Input: part model. Units: mm. Frame: model coordinates. A direction names the side the tool comes from. Round coordinates to 2 decimals unless told otherwise and drop trailing zeros. Loops run counter-clockwise (first coordinate to the right, second up) from the corner with the lowest first, then second, coordinate; pieces in that order, holes last. Notation, with made-up numbers: (-29, 36.5) - (-2, 36.5) arc R30 ccw to (-2, 58.5) - close; hole circle Ø6 at (82.5, 34.5). An arc over 180 degrees is marked (long way). One line per question, with ' | ' between items. Start each with the question number.
Item 1: Draft query along X for faces 4 (the face through (20, 23.85, -20)), 5 (the face through (-12.5, 14, 0)), 6 (the face through (18.134, 13.942, -35.15)). Return one class per face: pulls with the +X half, pulls with the -X half, needs draft (parallel to the pull), parting line crosses it, or undercut.
Item 2: Set-up query: faces 1 (the face through (0, 23.85, 0)), 2 (the face through (26.812, 13.609, -12.528)), 3 (the face through (13, 14, -12)). Return all of +Z, -Z, +X, -X, +Y, -Y with unobstructed straight access to the full face (end or side cutting, diameter ignored); none if empty.
Item 3: First-contact query: pin 1 (6 mm diameter, centred on x = 1.5, z = -1, fed in from -Y); pin 2 (6 mm diameter, centred on y = 16, z = -17.5, fed in from -X); pin 3 (12 mm diameter, centred on x = 23.5, y = 23.5, fed in from +Z). Flat tips, straight axial feed; report the tip coordinate or a pass-through.
Item 4: Section B-B, the plane x = -3. Return loops of the section in (y, z), plus the area to 3 significant figures.
Item 5: Section A-A, the plane y = 15.75. Return loops of the section in (x, z), plus the area to 3 significant figures.
Item 6: Section D-D, the plane z = -11.5. Return loops of the section in (x, y).
Item 7: Section C-C, the plane z = -1.5. Return loops of the section in (x, y).
Item 8: Material intervals for line 1 along Z through (x, y) = (8.5, 5.75); line 2 along X through (y, z) = (18.25, -6); line 3 along X through (y, z) = (7.75, 2), sorted ascending.
```python
from build123d import *

# Parameters (mm, degrees)
SKETCH_1_W           = 25
SKETCH_1_H           = 25
SKETCH_1_W_2         = 20.2
SKETCH_1_H_2         = 20.2
EXTRUDE_1_DEPTH      = 20
SKETCH_2_W           = 25
SKETCH_2_H           = 25
EXTRUDE_2_DEPTH      = 7.5
EXTRUDE_3_DEPTH      = 17.67767
EXTRUDE_3_DEPTH_BACK = 20
SKETCH_3_W           = 35.35533906
SKETCH_3_H           = 27.5
SKETCH_3_W_2         = 20.2
SKETCH_3_H_2         = 20.2
SKETCH_1_3_W         = 20.2
SKETCH_1_3_H         = 20.2
CUT_EXTRUDE_1_DEPTH  = 23.85
SKETCH_3_2_W         = 20.2
SKETCH_3_2_H         = 20.2
CUT_EXTRUDE_2_DEPTH  = 20
EXTRUDE_4_REACH      = 62.275


with BuildPart() as part:
    # 스케치1 → 보스-돌출1 (new body)
    with BuildSketch(Plane(origin=(0, 0, 0), x_dir=(1, 0, 0), z_dir=(0, 1, 0))):
        Rectangle(SKETCH_1_W, SKETCH_1_H)
        Rectangle(SKETCH_1_W_2, SKETCH_1_H_2, mode=Mode.SUBTRACT)
    extrude(amount=EXTRUDE_1_DEPTH)

    # 스케치2 → 보스-돌출2 (add)
    with BuildSketch(Plane(origin=(0, 20, 0), x_dir=(1, 0, 0), z_dir=(0, 1, 0))):
        Rectangle(SKETCH_2_W, SKETCH_2_H)
    extrude(amount=EXTRUDE_2_DEPTH)

    # 스케치3 → 보스-돌출3 (add, two sides: drawn at the far end of the back side and taken through both)
    with BuildSketch(Plane(origin=(12.5, 0, -12.5), x_dir=(0.7071067811865476, 0, 0.7071067811865476), z_dir=(-0.7071067811865476, 0, 0.7071067811865476)).offset(-EXTRUDE_3_DEPTH_BACK)):
        with Locations((0, 13.75)):
            Rectangle(SKETCH_3_W, SKETCH_3_H)
        with Locations((0, 13.75)):
            Rectangle(SKETCH_3_W_2, SKETCH_3_H_2, mode=Mode.SUBTRACT)
    extrude(amount=EXTRUDE_3_DEPTH + EXTRUDE_3_DEPTH_BACK)

    # 스케치1<3> → 컷-돌출1 (cut)
    with BuildSketch(Plane(origin=(0, 0, 0), x_dir=(1, 0, 0), z_dir=(0, 1, 0))):
        Rectangle(SKETCH_1_3_W, SKETCH_1_3_H)
    extrude(amount=CUT_EXTRUDE_1_DEPTH, mode=Mode.SUBTRACT)

    # 스케치3<2> → 컷-돌출2 (cut)
    with BuildSketch(Plane(origin=(12.5, 0, -12.5), x_dir=(0.7071067811865476, 0, 0.7071067811865476), z_dir=(-0.7071067811865476, 0, 0.7071067811865476))):
        with Locations((0, 13.75)):
            Rectangle(SKETCH_3_2_W, SKETCH_3_2_H)
    extrude(amount=CUT_EXTRUDE_2_DEPTH, mode=Mode.SUBTRACT)

    # 스케치5 → 보스-돌출4 (add, up to next)
    with BuildSketch(Plane(origin=(0, 3.65, 0), x_dir=(1, 0, 0), z_dir=(0, 1, 0)), mode=Mode.PRIVATE) as extrude_4_sk1:
        Polygon((19.64177849, 5.35822151), (5.35822151, 19.64177849), (-4.18355698, 10.1), (10.1, 10.1), (10.1, -4.18355698), align=None)
    extrude_4_tool1 = extrude(extrude_4_sk1.sketch, amount=EXTRUDE_4_REACH, mode=Mode.PRIVATE) - part.part
    add(extrude_4_tool1.solids().sort_by_distance((12.261747, 3.65, -12.261747))[0])


solid = part.part
```
Return value:
1) face 4: undercut | face 5: pulls with the -X half | face 6: pulls with the +X half
2) face 1: -Y | face 2: -Z | face 3: none
3) pin 1: y = 23.85 | pin 2: x = -10.5 | pin 3: z = 7.5
4) outline: (0, -22) - (27.5, -22) - (27.5, 12.5) - (0, 12.5) - (0, 10.1) - (23.85, 10.1) - (23.85, -10.1) - (0, -10.1) - close | area: 467 mm2
5) outline: (-12.5, -12.5) - (14.14, -39.14) - (19.5, -33.78) - (5.36, -19.64) - (19.64, -5.36) - (33.78, -19.5) - (39.14, -14.14) - (12.5, 12.5) - (-12.5, 12.5) - close; hole (-10.1, -10.1) - (10.1, -10.1) - (10.1, 10.1) - (-10.1, 10.1) - close | area: 833 mm2
6) outline: (-12.5, 0) - (36.5, 0) - (36.5, 27.5) - (-12.5, 27.5) - close; hole (13.5, 3.65) - (25.78, 3.65) - (25.78, 23.85) - (13.5, 23.85) - close
7) outline: (-12.5, 0) - (-10.1, 0) - (-10.1, 23.85) - (10.1, 23.85) - (10.1, 0) - (26.5, 0) - (26.5, 27.5) - (-12.5, 27.5) - close
8) line 1: -33.5 to -22.78, -16.5 to -10.1, 10.1 to 12.5 | line 2: -12.5 to -10.1, 10.1 to 19, 20.28 to 31 | line 3: -12.5 to -10.1, 10.1 to 23
